Design review of the part built by this model. Coordinates are the model's own, in mm. Face numbers are marked on the shaded views. A direction names the side the tool comes from. Coordinates: 2 decimals unless noted, no trailing zeros. Write each loop counter-clockwise with the first axis right and the second up, starting at its lowest first coordinate (ties: lowest second). Pieces come first, ordered by that corner, then holes. Notation, with made-up numbers: (22, -18.5) - (71, -18.5) arc R20 ccw to (71, -10.5) - close; hole circle Ø7 at (12, 62). An arc over 180 degrees is marked (long way). One line per item, written item: value.
Autodesk Inventor part; units mm, degrees
ref_plane "YZ Plane" through (0, 0, 0) normal (1, 0, 0) x (0, 1, 0)
ref_plane "XZ Plane" through (0, 0, 0) normal (0, 1, 0) x (-1, 0, 0)
ref_plane "XY Plane" through (0, 0, 0) normal (0, 0, 1) x (1, 0, 0)
sketch "Эскиз1" plane through (0, 0, 0) normal (0, 0, 1) x (1, 0, 0)
  point P0 (0, 0)
sketch "Эскиз2" plane through (0, 0, 0) normal (1, 0, 0) x (0, 1, 0)
  line L0 (54.4194, 8.3986) -> (39.8994, 8.3986)
  line L1 (59.4094, -4.1014) -> (59.4094, 3.8986)
  line L2 (64.4094, 15.8986) -> (64.4094, -11.1014)
  line L3 (61.9094, 18.3986) -> (34.9094, 18.3986)
  line L4 (32.4094, 20.8986) -> (32.4094, 47.8986)
  line L5 (23.4094, 30.3986) -> (6.4094, 30.3986)
  line L6 (27.4094, 14.7056) -> (27.4094, 16.0719)
  line L7 (59.4094, -11.1014) -> (64.4094, -11.1014)
  line L8 (64.4094, -11.1014) -> (64.4094, 18.3986)
  line L9 (64.4094, 18.3986) -> (59.4094, 18.3986)
  line L10 (59.4094, 18.3986) -> (59.4094, -11.1014)
  line L11 (32.4094, 8.3986) -> (59.4094, 8.3986)
  line L12 (59.4094, 8.3986) -> (59.4094, 18.3986)
  line L13 (59.4094, 18.3986) -> (32.4094, 18.3986)
  line L14 (32.4094, 18.3986) -> (32.4094, 8.3986)
  line L15 (27.4094, 8.3986) -> (32.4094, 8.3986)
  line L16 (32.4094, 8.3986) -> (32.4094, 47.8986)
  line L17 (32.4094, 47.8986) -> (27.4094, 47.8986)
  line L18 (27.4094, 47.8986) -> (27.4094, 8.3986)
  line L19 (6.4094, 30.3986) -> (27.4094, 30.3986)
  line L20 (27.4094, 30.3986) -> (27.4094, 47.8986)
  line L21 (27.4094, 47.8986) -> (6.4094, 47.8986)
  line L22 (6.4094, 47.8986) -> (6.4094, 30.3986)
  point P0 (0, 0)
  point P1 (59.4094, 8.3986)
  point P2 (61.9094, 18.3986)
  point P3 (34.9094, 18.3986)
  point P4 (32.4094, 8.3986)
  point P5 (27.4094, 8.3986)
extrude "Выдавливание1" add sketch "Эскиз2" along normal mid plane 150
sketch "Эскиз3" plane through (75, 59.4094, 8.3986) normal (0, 0, -1) x (-1, 0, 0)
  circle A0 centre (147, -11) radius 1.85
  circle A1 centre (3, -11) radius 1.85
  circle A2 centre (11, -19) radius 1.85
  circle A3 centre (139, -19) radius 1.85
  point P0 (75, -59.4094)
extrude "Выдавливание2" cut sketch "Эскиз3" against normal through all
sketch "Эскиз4" plane through (75, 59.4094, 8.3986) normal (0, 0, -1) x (-1, 0, 0)
  line L0 (150, 0) -> (150, -32)
  line L1 (150, 0) -> (0, 0)
  line L2 (150, -32) -> (129.5965, -32)
  line L3 (129.5965, -32) -> (129.5965, 0)
  line L4 (129.5965, 0) -> (150, 0)
  line L5 (150, 0) -> (150, -32)
  line L6 (150, -32) -> (0, -32)
  point P0 (75, -59.4094)
  point P1 (139.7982, -32)
extrude "Выдавливание3" cut sketch "Эскиз4" against normal blind 5
mirror "Зеркальное отражение1" about plane through (0, 0, 0) normal (1, 0, 0) of "Выдавливание3"
sketch "Эскиз5" plane through (-75, 6.4094, 47.8986) normal (0, 0, 1) x (1, 0, 0)
  circle A0 centre (97.5, 8.5) radius 1.25
  circle A1 centre (52.5, 8.5) radius 1.25
  circle A2 centre (100, 40.75) radius 1.2645
  circle A3 centre (50, 40.75) radius 1.2645
  point P0 (75, -6.4094)
extrude "Выдавливание4" cut sketch "Эскиз5" against normal through all
sketch "Эскиз6" plane through (-75, 6.4094, 47.8986) normal (0, 0, 1) x (1, 0, 0)
  circle A0 centre (97.5, 8.5) radius 1.25
  circle A1 centre (97.5, 8.5) radius 5
  circle A2 centre (52.5, 8.5) radius 1.25
  circle A3 centre (52.5, 8.5) radius 5
  point P0 (75, -6.4094)
  dimension "d8" = 10
  dimension "d9" = 10
extrude "Выдавливание5" cut sketch "Эскиз6" against normal blind 14.5 contours A0 | A1 | A2 | A3
sketch "Эскиз7" plane through (-75, 32.4094, 18.3986) normal (0, 0, 1) x (1, 0, 0)
  circle A0 centre (100, 14.75) radius 1.2645
  circle A1 centre (100, 14.75) radius 5
  circle A2 centre (50, 14.75) radius 1.2645
  circle A3 centre (50, 14.75) radius 5
  point P0 (75, -32.4094)
  dimension "d12" = 10
  dimension "d13" = 10
extrude "Выдавливание6" cut sketch "Эскиз7" against normal blind 7 contours A0 | A1 | A2 | A3
fillet "Сопряжение1" radius 21 2 edges at (75, 6.4094, 39.1486) (-75, 6.4094, 39.1486)
chamfer "Фаска1" distance 5 angle 45 2 edges at (64.7982, 59.4094, 13.3986) (-64.7982, 59.4094, 13.3986)
chamfer "Фаска2" distance 5 angle 45 1 edges at (0, 27.4094, 8.3986)
properties part number "000.001.010 - Realsense крепление"
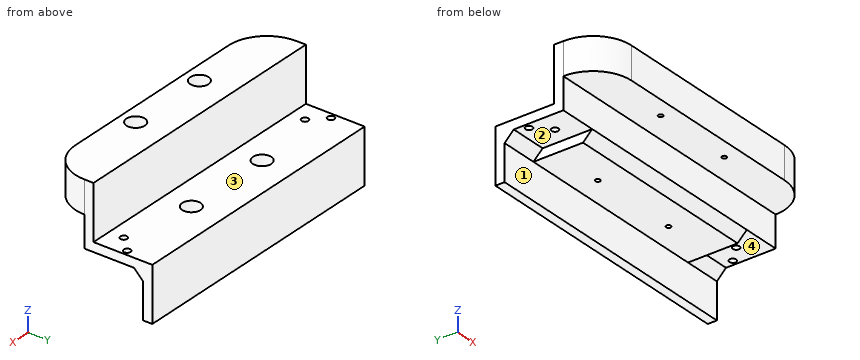
1. Consider section A-A, the plane x = 0. Write out the cut boundary in (y, z), then the cut area to 3 significant figures.
Answer block:
outline: (6.41, 30.4) - (27.41, 30.4) - (27.41, 13.4) - (32.41, 8.4) - (59.41, 8.4) - (59.41, -11.1) - (64.41, -11.1) - (64.41, 18.4) - (32.41, 18.4) - (32.41, 47.9) - (6.41, 47.9) - close
area: 970 mm^2
2. Consider section B-B, the plane x = 72. Write out the cut boundary in (y, z).
Answer block:
outline: (16.59, 30.4) - (27.41, 30.4) - (27.41, 13.4) - (46.56, 13.4) - (46.56, 18.4) - (32.41, 18.4) - (32.41, 47.9) - (16.59, 47.9) - close; (50.26, 13.4) - (54.41, 13.4) - (59.41, 8.4) - (59.41, -11.1) - (64.41, -11.1) - (64.41, 18.4) - (50.26, 18.4) - close
3. For the marked faces 1, 2, 3 and 4, list the 3-axis set-ups (+Z, -Z, +X, -X, +Y, -Y) from which the entire face can be reached by the end or side of a thin tool; tool diameter is ignored.
Answer block:
face 1: -Z, +X, -X, -Y
face 2: -Z, -X, -Y
face 3: +Z, +X, -X, +Y
face 4: -Z, +X, -Y
4. Consider section D-D, the plane z = 41. Write out the cut boundary in (x, y).
Answer block:
outline: (-75, 27.41) arc R21 ccw to (-54, 6.41) - (54, 6.41) arc R21 ccw to (75, 27.41) - (75, 32.41) - (-75, 32.41) - close; hole circle Ø10 at (-22.5, 14.91); hole circle Ø10 at (22.5, 14.91)
5. Insertion check: pin 1 Ø10 at (x, y) = (66, 40.5) entering from -Z; pin 2 Ø1.5 at (x, z) = (30.5, 4) entering from -Y; pin 3 Ø9.5 at (x, y) = (35.5, 43.5) entering from +Z; pin 4 Ø2 at (x, y) = (64, 40.41) entering from +Z. Each pin has a flat end and moves straight along its axis. Give the tip position at first contact, or say it passes through.
Answer block:
pin 1: stops at z = 13.4
pin 2: stops at y = 59.41
pin 3: stops at z = 18.4
pin 4: passes through
6. Consider section C-C, the plane y = 37. Write out the cut boundary in (x, z), then the cut area to 3 significant figures.
Answer block:
outline: (-75, 13.4) - (-54.6, 13.4) - (-54.6, 8.4) - (54.6, 8.4) - (54.6, 13.4) - (75, 13.4) - (75, 18.4) - (-75, 18.4) - close
area: 1,300 mm^2
7. Wall thickness on line 1 along Y through (x, z) = (-64, 16.45); line 2 along Y through (x, z) = (22.5, 31.35); line 3 along Y through (x, z) = (-11, 38): over which ranges is each line inside the solid? List them lowest first.
Answer block:
line 1: y = 27.41 to 38.56, 42.26 to 64.41
line 2: y = 6.41 to 13.66, 16.16 to 32.41
line 3: y = 6.41 to 32.41
